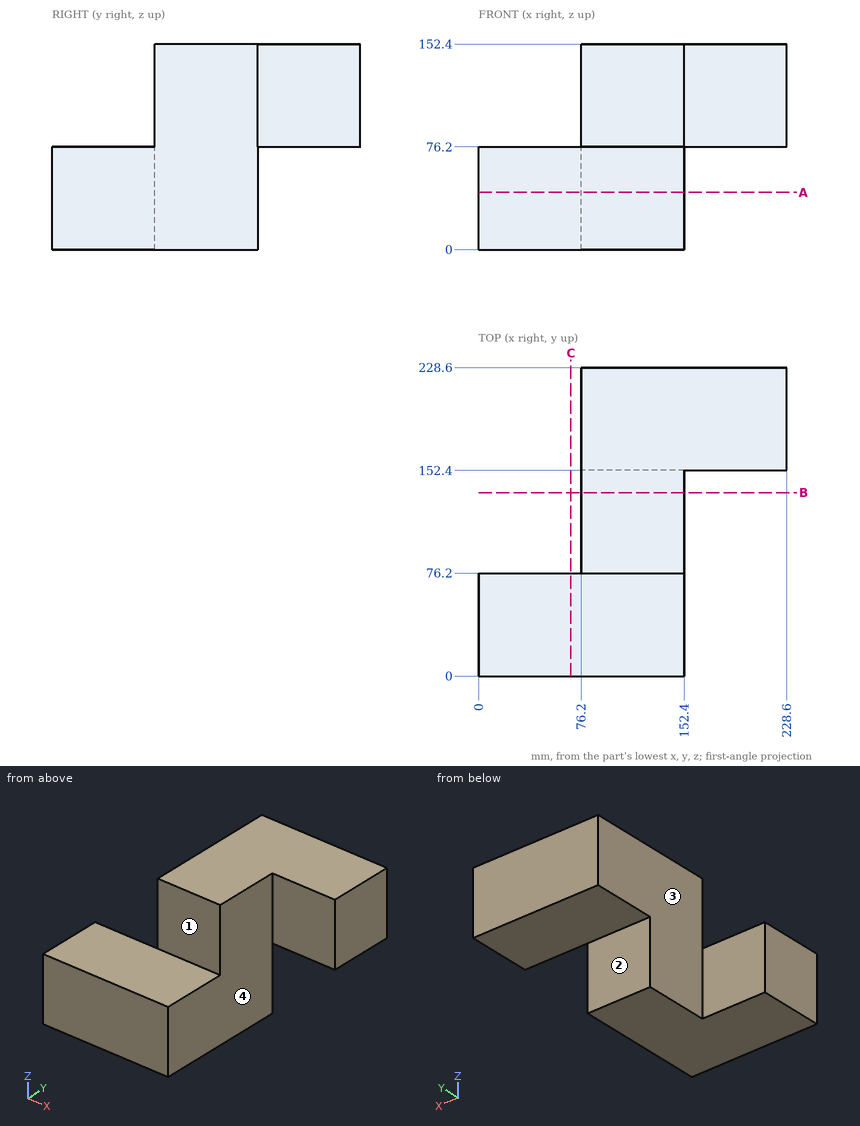
For this review, use the dimensioned drawing (mm, ordinates from the lowest corner) and the shaded views. A direction names the side the tool comes from. Coordinates: 2 decimals unless noted, no trailing zeros. Write each loop counter-clockwise with the first axis right and the second up, starting at its lowest first coordinate (ties: lowest second). Pieces come first, ordered by that corner, then holes. Notation, with made-up numbers: (-37.5, -17.5) - (-9.5, -17.5) arc R28 ccw to (-9.5, 3.5) - close; hole circle Ø6 at (64.5, -29). An arc over 180 degrees is marked (long way). One line per item, written item: value.
1) For the marked faces 1, 2, 3 and 4, list the 3-axis set-ups (+Z, -Z, +X, -X, +Y, -Y) from which the entire face can be reached by the end or side of a thin tool; tool diameter is ignored.
Answer sheet:
face 1: +Z, +X, -X, -Y
face 2: -Z, +X, -X, +Y
face 3: +Z, -Z, -X, +Y
face 4: +Z, -Z, +X, -Y
2) Add section C-C (x = 68.5). State the section outline as (y, z) points, plus the area to 3 significant figures.
Answer sheet:
outline: (0, 0) - (76.2, 0) - (76.2, 76.2) - (0, 76.2) - close
area: 5,810 mm2
3) Add section A-A (z = 42.5). State the section outline as (x, y) points.
Answer sheet:
outline: (0, 0) - (152.4, 0) - (152.4, 152.4) - (76.2, 152.4) - (76.2, 76.2) - (0, 76.2) - close
4) To check wall thickness, follow probe 1 along X at (y, z) = (80, 100.5); probe 2 along X at (y, z) = (166, 126.5); probe 3 along Z at (x, y) = (146.5, 13). State the ranges of each line that lie inside material, in increasing order.
Answer sheet:
probe 1: x = 76.2 to 152.4
probe 2: x = 76.2 to 228.6
probe 3: z = 0 to 76.2
5) Insertion check: pin 1 (8 mm diameter, centred on y = 113, z = 18.5, fed in from +X); pin 2 (6 mm diameter, centred on x = 120, z = 40, fed in from +Y); pin 3 (1 mm diameter, centred on x = 101, y = 36, fed in from +Z). Each pin has a flat end and moves straight along its axis. Give the tip position at first contact, or say it passes through.
Answer sheet:
pin 1: stops at x = 152.4
pin 2: stops at y = 152.4
pin 3: stops at z = 76.2
6) Add section B-B (y = 136). State the section outline as (x, z) points, plus the area to 3 significant figures.
Answer sheet:
outline: (76.2, 0) - (152.4, 0) - (152.4, 152.4) - (76.2, 152.4) - close
area: 11,600 mm2
